Input: part model. Units: mm. Frame: model coordinates. A direction names the side the tool comes from. Coordinates: 2 decimals unless noted, no trailing zeros. Order: outer loops, then holes, each group sorted by start corner. A loop starts at its lowest first (then second) coordinate and runs counter-clockwise, first axis right, second up. Notation, with made-up numbers: M -2.75,-13.5 L 14.25,-13.5 A10 ccw 14.25,-3.5 Z; hole C -1.5,15.5 d9. An arc over 180 degrees is marked long. Answer in a Markdown table with one row per item.
from build123d import *

# Parameters (mm, degrees)
SKETCH1_W               = 30
SKETCH1_H               = 30
BOSS_EXTRUDE3_DEPTH     = 95
BOSS_EXTRUDE4_DEPTH     = 30
CUT_EXTRUDE1_DEPTH      = 147.287388383
SKETCH5_R               = 10
BOSS_EXTRUDE5_DEPTH     = 5.71
SKETCH6_R               = 8.4
BOSS_EXTRUDE6_DEPTH     = 30
SKETCH8_R               = 1.5
SKETCH8_R_2             = 2.5
CUT_EXTRUDE2_DEPTH      = 158.536675412
CHAMFER1_SIZE           = 1.5
CHAMFER2_SIZE           = 3.5
CUT_EXTRUDE3_DEPTH      = 17
CUT_EXTRUDE4_DEPTH      = 10
CUT_EXTRUDE4_DEPTH_BACK = 2
SKETCH10_W              = 14.270411079
SKETCH10_H              = 4.897722898


with BuildPart() as part:
    # Sketch1 → Boss-Extrude3 (new body)
    with BuildSketch(Plane.XY):
        with Locations((15, 15)):
            Rectangle(SKETCH1_W, SKETCH1_H)
        with BuildLine():
            Line((17.802943725, 19.5), (12.197056275, 19.5))
            Line((12.197056275, 19.5), (10.289949494, 21.407106781))
            Line((10.289949494, 21.407106781), (10.289949494, 22.7))
            Line((10.289949494, 22.7), (11.517157288, 22.7))
            ThreePointArc((11.517157288, 22.7), (12.16387296, 23.132121597), (12.012132034, 23.894974747))
            Line((12.012132034, 23.894974747), (10.612132034, 25.294974747))
            Line((10.612132034, 25.294974747), (4.705025253, 25.294974747))
            Line((4.705025253, 25.294974747), (4.705025253, 19.387867966))
            Line((4.705025253, 19.387867966), (6.105025253, 17.987867966))
            ThreePointArc((6.105025253, 17.987867966), (6.867878403, 17.83612704), (7.3, 18.482842712))
            Line((7.3, 18.482842712), (7.3, 19.710050506))
            Line((7.3, 19.710050506), (8.592893219, 19.710050506))
            Line((8.592893219, 19.710050506), (10.5, 17.802943725))
            Line((10.5, 17.802943725), (10.5, 12.197056275))
            Line((10.5, 12.197056275), (8.592893219, 10.289949494))
            Line((8.592893219, 10.289949494), (7.3, 10.289949494))
            Line((7.3, 10.289949494), (7.3, 11.517157288))
            ThreePointArc((7.3, 11.517157288), (6.867878403, 12.16387296), (6.105025253, 12.012132034))
            Line((6.105025253, 12.012132034), (4.705025253, 10.612132034))
            Line((4.705025253, 10.612132034), (4.705025253, 4.705025253))
            Line((4.705025253, 4.705025253), (10.612132034, 4.705025253))
            Line((10.612132034, 4.705025253), (12.012132034, 6.105025253))
            ThreePointArc((12.012132034, 6.105025253), (12.16387296, 6.867878403), (11.517157288, 7.3))
            Line((11.517157288, 7.3), (10.289949494, 7.3))
            Line((10.289949494, 7.3), (10.289949494, 8.592893219))
            Line((10.289949494, 8.592893219), (12.197056275, 10.5))
            Line((12.197056275, 10.5), (17.802943725, 10.5))
            Line((17.802943725, 10.5), (19.710050506, 8.592893219))
            Line((19.710050506, 8.592893219), (19.710050506, 7.3))
            Line((19.710050506, 7.3), (18.482842712, 7.3))
            ThreePointArc((18.482842712, 7.3), (17.83612704, 6.867878403), (17.987867966, 6.105025253))
            Line((17.987867966, 6.105025253), (19.387867966, 4.705025253))
            Line((19.387867966, 4.705025253), (25.294974747, 4.705025253))
            Line((25.294974747, 4.705025253), (25.294974747, 10.612132034))
            Line((25.294974747, 10.612132034), (23.894974747, 12.012132034))
            ThreePointArc((23.894974747, 12.012132034), (23.132121597, 12.16387296), (22.7, 11.517157288))
            Line((22.7, 11.517157288), (22.7, 10.289949494))
            Line((22.7, 10.289949494), (21.407106781, 10.289949494))
            Line((21.407106781, 10.289949494), (19.5, 12.197056275))
            Line((19.5, 12.197056275), (19.5, 17.802943725))
            Line((19.5, 17.802943725), (21.407106781, 19.710050506))
            Line((21.407106781, 19.710050506), (22.7, 19.710050506))
            Line((22.7, 19.710050506), (22.7, 18.482842712))
            ThreePointArc((22.7, 18.482842712), (23.132121597, 17.83612704), (23.894974747, 17.987867966))
            Line((23.894974747, 17.987867966), (25.294974747, 19.387867966))
            Line((25.294974747, 19.387867966), (25.294974747, 25.294974747))
            Line((25.294974747, 25.294974747), (19.387867966, 25.294974747))
            Line((19.387867966, 25.294974747), (17.987867966, 23.894974747))
            ThreePointArc((17.987867966, 23.894974747), (17.83612704, 23.132121597), (18.482842712, 22.7))
            Line((18.482842712, 22.7), (19.710050506, 22.7))
            Line((19.710050506, 22.7), (19.710050506, 21.407106781))
            Line((19.710050506, 21.407106781), (17.802943725, 19.5))
        make_face(mode=Mode.SUBTRACT)
    extrude(amount=BOSS_EXTRUDE3_DEPTH)

    # Sketch3 → Boss-Extrude4 (add)
    with BuildSketch(Plane(origin=(30, 0, 0), x_dir=(0, 0, -1), z_dir=(1, 0, 0))):
        with BuildLine():
            Line((-125, 30), (-95, 30))
            Line((-95, 30), (-95, 0))
            Line((-95, 0), (-125, 0))
            ThreePointArc((-125, 0), (-140, 15), (-125, 30))
        make_face()
    extrude(amount=-BOSS_EXTRUDE4_DEPTH)

    # Sketch4 → Cut-Extrude1 (cut, through all)
    with BuildSketch(Plane(origin=(0, 30, 0), x_dir=(1, 0, 0), z_dir=(0, 1, 0))):
        with BuildLine():
            Line((5, -97.729588921), (13.490616116, -97.729588921))
            ThreePointArc((13.490616116, -97.729588921), (17.026150022, -99.194055015), (18.490616116, -102.729588921))
            Line((18.490616116, -102.729588921), (18.490616116, -140))
            Line((18.490616116, -140), (0, -140))
            Line((0, -140), (0, -92.729588921))
            ThreePointArc((0, -92.729588921), (1.464466094, -96.265122827), (5, -97.729588921))
        make_face()
    extrude(amount=-CUT_EXTRUDE1_DEPTH, mode=Mode.SUBTRACT)

    # Sketch5 → Boss-Extrude5 (add)
    with BuildSketch(Plane(origin=(30, 0, 0), x_dir=(0, 0, -1), z_dir=(1, 0, 0))):
        with Locations(Location((-125, 15, 0), (0, 0, 180))):
            Circle(SKETCH5_R)
    extrude(amount=BOSS_EXTRUDE5_DEPTH)

    # Sketch6 → Boss-Extrude6 (add)
    with BuildSketch(Plane(origin=(35.71, 0, 0), x_dir=(0, 0, -1), z_dir=(1, 0, 0))):
        with Locations((-125, 15)):
            Circle(SKETCH6_R)
    extrude(amount=BOSS_EXTRUDE6_DEPTH)

    # Sketch8 → Cut-Extrude2 (cut, through all)
    with BuildSketch(Plane.ZY):
        with Locations((6.7, 15)):
            Circle(SKETCH8_R)
        with Locations((86.4, 15)):
            Circle(SKETCH8_R)
        with Locations((28.8, 15)):
            Circle(SKETCH8_R_2)
        with Locations((125, 15)):
            Circle(SKETCH8_R_2)
    extrude(amount=-CUT_EXTRUDE2_DEPTH, mode=Mode.SUBTRACT)

    # Chamfer1
    chamfer1_edges = [part.edges().sort_by_distance(p)[0] for p in [
        (30, 15, 140),
        (18.490616116, 15, 140),
        (0, 30, 46.364794461),
        (0, 0, 46.364794461),
        (18.490616116, 30, 113.864794461),
        (17.026150022, 30, 99.194055015),
        (9.245308058, 30, 97.729588921),
        (1.464466094, 30, 96.265122827),
        (18.490616116, 0, 113.864794461),
        (1.464466094, 0, 96.265122827),
        (9.245308058, 0, 97.729588921),
        (17.026150022, 0, 99.194055015),
        (30, 30, 62.5),
        (30, 0, 62.5),
    ]]
    chamfer(chamfer1_edges, length=CHAMFER1_SIZE)

    # Chamfer2
    chamfer2_edges = [part.edges().sort_by_distance(p)[0] for p in [
        (30, 15, 115),
    ]]
    chamfer(chamfer2_edges, length=CHAMFER2_SIZE - 0.0001)  # a hair under: the kernel refuses the full size

    # Sketch9 → Cut-Extrude3 (cut)
    with BuildSketch(Plane(origin=(0, 0, 95), x_dir=(-1, 0, 0), z_dir=(0, 0, -1))):
        with BuildLine():
            Line((-10.612132034, 4.705025253), (-4.705025253, 4.705025253))
            Line((-4.705025253, 4.705025253), (-4.705025253, 10.612132034))
            Line((-4.705025253, 10.612132034), (-6.105025253, 12.012132034))
            ThreePointArc((-6.105025253, 12.012132034), (-6.867878403, 12.16387296), (-7.3, 11.517157288))
            Line((-7.3, 11.517157288), (-7.3, 10.289949494))
            Line((-7.3, 10.289949494), (-8.592893219, 10.289949494))
            Line((-8.592893219, 10.289949494), (-10.5, 12.197056275))
            Line((-10.5, 12.197056275), (-10.5, 17.802943725))
            Line((-10.5, 17.802943725), (-8.592893219, 19.710050506))
            Line((-8.592893219, 19.710050506), (-7.3, 19.710050506))
            Line((-7.3, 19.710050506), (-7.3, 18.482842712))
            ThreePointArc((-7.3, 18.482842712), (-6.867878403, 17.83612704), (-6.105025253, 17.987867966))
            Line((-6.105025253, 17.987867966), (-4.705025253, 19.387867966))
            Line((-4.705025253, 19.387867966), (-4.705025253, 25.294974747))
            Line((-4.705025253, 25.294974747), (-10.612132034, 25.294974747))
            Line((-10.612132034, 25.294974747), (-12.012132034, 23.894974747))
            ThreePointArc((-12.012132034, 23.894974747), (-12.16387296, 23.132121597), (-11.517157288, 22.7))
            Line((-11.517157288, 22.7), (-10.289949494, 22.7))
            Line((-10.289949494, 22.7), (-10.289949494, 21.407106781))
            Line((-10.289949494, 21.407106781), (-12.197056275, 19.5))
            Line((-12.197056275, 19.5), (-17.802943725, 19.5))
            Line((-17.802943725, 19.5), (-19.710050506, 21.407106781))
            Line((-19.710050506, 21.407106781), (-19.710050506, 22.7))
            Line((-19.710050506, 22.7), (-18.482842712, 22.7))
            ThreePointArc((-18.482842712, 22.7), (-17.83612704, 23.132121597), (-17.987867966, 23.894974747))
            Line((-17.987867966, 23.894974747), (-19.387867966, 25.294974747))
            Line((-19.387867966, 25.294974747), (-25.294974747, 25.294974747))
            Line((-25.294974747, 25.294974747), (-25.294974747, 19.387867966))
            Line((-25.294974747, 19.387867966), (-23.894974747, 17.987867966))
            ThreePointArc((-23.894974747, 17.987867966), (-23.132121597, 17.83612704), (-22.7, 18.482842712))
            Line((-22.7, 18.482842712), (-22.7, 19.710050506))
            Line((-22.7, 19.710050506), (-21.407106781, 19.710050506))
            Line((-21.407106781, 19.710050506), (-19.5, 17.802943725))
            Line((-19.5, 17.802943725), (-19.5, 12.197056275))
            Line((-19.5, 12.197056275), (-21.407106781, 10.289949494))
            Line((-21.407106781, 10.289949494), (-22.7, 10.289949494))
            Line((-22.7, 10.289949494), (-22.7, 11.517157288))
            ThreePointArc((-22.7, 11.517157288), (-23.132121597, 12.16387296), (-23.894974747, 12.012132034))
            Line((-23.894974747, 12.012132034), (-25.294974747, 10.612132034))
            Line((-25.294974747, 10.612132034), (-25.294974747, 4.705025253))
            Line((-25.294974747, 4.705025253), (-19.387867966, 4.705025253))
            Line((-19.387867966, 4.705025253), (-17.987867966, 6.105025253))
            ThreePointArc((-17.987867966, 6.105025253), (-17.83612704, 6.867878403), (-18.482842712, 7.3))
            Line((-18.482842712, 7.3), (-19.710050506, 7.3))
            Line((-19.710050506, 7.3), (-19.710050506, 8.592893219))
            Line((-19.710050506, 8.592893219), (-17.802943725, 10.5))
            Line((-17.802943725, 10.5), (-12.197056275, 10.5))
            Line((-12.197056275, 10.5), (-10.289949494, 8.592893219))
            Line((-10.289949494, 8.592893219), (-10.289949494, 7.3))
            Line((-10.289949494, 7.3), (-11.517157288, 7.3))
            ThreePointArc((-11.517157288, 7.3), (-12.16387296, 6.867878403), (-12.012132034, 6.105025253))
            Line((-12.012132034, 6.105025253), (-10.612132034, 4.705025253))
        make_face()
    extrude(amount=-CUT_EXTRUDE3_DEPTH, mode=Mode.SUBTRACT)

    # Sketch10 → Cut-Extrude4 (cut, two sides: drawn at the far end of the back side and taken through both)
    with BuildSketch(Plane.ZY.offset(-18.490616116).offset(-CUT_EXTRUDE4_DEPTH_BACK)):
        with Locations((104.864794461, 21.948861449)):
            Rectangle(SKETCH10_W, SKETCH10_H)
        with Locations((104.864794461, 8.051138551)):
            Rectangle(SKETCH10_W, SKETCH10_H)
    extrude(amount=CUT_EXTRUDE4_DEPTH + CUT_EXTRUDE4_DEPTH_BACK, mode=Mode.SUBTRACT)


solid = part.part
1) Cut plane B-B, the plane x = 41. Output: boundary loops of the cut face in (y, z).
Resolved:
| item | result |
|---|---|
| outline | C 15,125 d16.8; hole C 15,125 d5 |
2) Mould query, pull axis Y, two halves, no side actions, for faces 1 (the face through (15, 30, 49)), 2 (the face through (5.18, 14.04, 31.11)), 3 (the face through (8, 4.705, 48)), 4 (the face through (18.491, 15, 120)). Classes: +Y half, -Y half, draft (parallel to the pull), parting line (faces both ways), or undercut.
Resolved:
| item | result |
|---|---|
| face 1 | +Y half |
| face 2 | undercut |
| face 3 | undercut |
| face 4 | draft |
3) Cut plane A-A, the plane y = 15. State how many separate pieces and enclosed holes the cut face has, and give its area (3 significant figures).
Resolved:
| item | result |
|---|---|
| separate pieces | 9 |
| enclosed holes | 0 |
| area | 2,680 mm2 |
4) Reachability of faces 5 (the face through (17.3, 5.602, 98.7)), 6 (the face through (10.5, 15, 48)), 7 (the face through (34.59, 8.24, 117.63)), 8 (the face through (25.295, 22, 55)), 9 (the face through (8, 15, 97.73)) from +Z, -Z, +X, -X, +Y, -Y: full face, straight path, thin tool, end or side. Return the list, or none.
Resolved:
| item | result |
|---|---|
| face 5 | +Z, -X |
| face 6 | +Z, -Z |
| face 7 | +X |
| face 8 | -Z |
| face 9 | +Z, -X, +Y, -Y |
5) Contact query for flat-ended pins moving along their axis: pin 1 (8 mm diameter, centred on y = 8, z = 122.5, fed in from -X); pin 2 (5 mm diameter, centred on y = 4, z = 79, fed in from +X); pin 3 (12 mm diameter, centred on x = 41, y = 15.5, fed in from -Z). Output: stop coordinate, or through.
Resolved:
| item | result |
|---|---|
| pin 1 | stops at x = 18.49 |
| pin 2 | stops at x = 30 |
| pin 3 | stops at z = 115 |
6) Material intervals for probe 1 along X at (y, z) = (22.25, 18.5); probe 2 along Y at (x, z) = (22.5, 6.7); probe 3 along X at (y, z) = (20.5, 36.5), sorted ascending.
Resolved:
| item | result |
|---|---|
| probe 1 | x = 0 to 4.71, 10.29 to 19.71, 25.29 to 30 |
| probe 2 | y = 0 to 4.71, 10.29 to 13.5, 16.5 to 19.71, 25.29 to 30 |
| probe 3 | x = 0 to 4.71, 11.2 to 18.8, 25.29 to 30 |
